Work out the finished part from the listing and answer in its coordinate system (mm). A direction names the side the tool comes from. Coordinates: 2 decimals unless noted, no trailing zeros. Loops run counter-clockwise (first coordinate to the right, second up) from the corner with the lowest first, then second, coordinate; pieces in that order, holes last. Notation, with made-up numbers: M 50.5,69 L 102.5,69 A14 ccw 102.5,93 Z; hole C -1,27 d8. An arc over 180 degrees is marked long. Write each question's results on one line, items separated by ' | '.
```python
from build123d import *

# Parameters (mm, degrees)
ESBO_O1_W                = 69
ESBO_O1_H                = 31.5
RESSALTO_EXTRUS_O1_DEPTH = 6
ESBO_O2_W                = 5
ESBO_O2_H                = 20
RESSALTO_EXTRUS_O2_DEPTH = 20
ESBO_O3_W                = 5
ESBO_O3_H                = 8
CORTE_EXTRUS_O1_DEPTH    = 11
ESBO_O4_W                = 4
ESBO_O4_H                = 31.5
RESSALTO_EXTRUS_O3_DEPTH = 20
ESBO_O5_W                = 16
ESBO_O5_H                = 8
CORTE_EXTRUS_O2_DEPTH    = 4
ESBO_O6_W                = 4
ESBO_O6_H                = 31.5
RESSALTO_EXTRUS_O4_DEPTH = 50
ESBO_O18_R               = 3.8
CORTE_EXTRUS_O3_DEPTH    = 4
ESBO_O19_R               = 5.8
CORTE_EXTRUS_O5_DEPTH    = 4
ESBO_O20_W               = 20
ESBO_O20_H               = 45
RESSALTO_EXTRUS_O9_DEPTH = 7
ESBO_O21_W               = 13
ESBO_O21_H               = 15
CORTE_EXTRUS_O6_DEPTH    = 7.7
ESBO_O22_W               = 13
ESBO_O22_H               = 20
CORTE_EXTRUS_O7_DEPTH    = 7.7
CORTE_EXTRUS_O9_DEPTH    = 3


with BuildPart() as part:
    # Esboço1 → Ressalto-extrusão1 (new body)
    with BuildSketch(Plane.XY):
        with Locations((-34.5, -15.931977108)):
            Rectangle(ESBO_O1_W, ESBO_O1_H)
    extrude(amount=RESSALTO_EXTRUS_O1_DEPTH)

    # Esboço2 → Ressalto-extrusão2 (add)
    with BuildSketch(Plane.XY.offset(6)):
        with Locations((-60, -21.681977108)):
            Rectangle(ESBO_O2_W, ESBO_O2_H)
    extrude(amount=RESSALTO_EXTRUS_O2_DEPTH)

    # Esboço3 → Corte-extrusão1 (cut)
    with BuildSketch(Plane.XY.offset(26)):
        with Locations((-60, -21.681977108)):
            Rectangle(ESBO_O3_W, ESBO_O3_H)
    extrude(amount=-CORTE_EXTRUS_O1_DEPTH, mode=Mode.SUBTRACT)

    # Esboço4 → Ressalto-extrusão3 (add)
    with BuildSketch(Plane.XY.offset(6)):
        with Locations((-52, -15.931977108)):
            Rectangle(ESBO_O4_W, ESBO_O4_H)
    extrude(amount=RESSALTO_EXTRUS_O3_DEPTH)

    # Esboço5 → Corte-extrusão2 (cut)
    with BuildSketch(Plane(origin=(-50, 0, 0), x_dir=(0, 0, -1), z_dir=(1, 0, 0))):
        with Locations((-14, -21.681977108)):
            Rectangle(ESBO_O5_W, ESBO_O5_H)
    extrude(amount=-CORTE_EXTRUS_O2_DEPTH, mode=Mode.SUBTRACT)

    # Esboço6 → Ressalto-extrusão4 (add)
    with BuildSketch(Plane(origin=(-50, 0, 0), x_dir=(0, 0, -1), z_dir=(1, 0, 0))):
        with Locations((-24, -15.931977108)):
            Rectangle(ESBO_O6_W, ESBO_O6_H)
    extrude(amount=RESSALTO_EXTRUS_O4_DEPTH)

    # Espelhar10: part across plane


with BuildPart() as part_1:
    add(part.part)
    add(part.part.mirror(Plane.ZX.offset(-0.181977108)))

    # Espelhar11: part across plane


with BuildPart() as part_2:
    add(part_1.part)
    add(part_1.part.mirror(Plane(origin=(0, 0, 0), x_dir=(0, 0, 1), z_dir=(1, 0, 0))))

    # Esboço18 → Corte-extrusão3 (cut)
    with BuildSketch(Plane.ZY.offset(54)):
        with Locations((16, -0.181977108)):
            Circle(ESBO_O18_R)
    extrude(amount=-CORTE_EXTRUS_O3_DEPTH, mode=Mode.SUBTRACT)

    # Esboço19 → Corte-extrusão5 (cut)
    with BuildSketch(Plane.XY.offset(26)):
        with Locations((35, 20.318022892)):
            Circle(ESBO_O19_R)
    extrude(amount=-CORTE_EXTRUS_O5_DEPTH, mode=Mode.SUBTRACT)

    # Esboço20 → Ressalto-extrusão9 (add)
    with BuildSketch(Plane(origin=(0, 0, 22), x_dir=(-1, 0, 0), z_dir=(0, 0, -1))):
        with Locations((34, -0.181977108)):
            Rectangle(ESBO_O20_W, ESBO_O20_H)
    extrude(amount=RESSALTO_EXTRUS_O9_DEPTH)

    # Esboço21 → Corte-extrusão6 (cut)
    with BuildSketch(Plane.XY.offset(26)):
        with Locations((-34, -12.181977108)):
            Rectangle(ESBO_O21_W, ESBO_O21_H)
    extrude(amount=-CORTE_EXTRUS_O6_DEPTH, mode=Mode.SUBTRACT)

    # Esboço22 → Corte-extrusão7 (cut)
    with BuildSketch(Plane.XY.offset(26)):
        with Locations((-34, 8.318022892)):
            Rectangle(ESBO_O22_W, ESBO_O22_H)
    extrude(amount=-CORTE_EXTRUS_O7_DEPTH, mode=Mode.SUBTRACT)

    # Esboço23 → Corte-extrusão9 (cut)
    with BuildSketch(Plane(origin=(0, -1.681977108, 0), x_dir=(1, 0, 0), z_dir=(0, 1, 0))):
        with BuildLine():
            Line((-31, -26), (-31, -22.15))
            ThreePointArc((-31, -22.15), (-34, -19.15), (-37, -22.15))
            Line((-37, -22.15), (-37, -26))
            Line((-37, -26), (-31, -26))
        make_face()
    extrude(amount=-CORTE_EXTRUS_O9_DEPTH, mode=Mode.SUBTRACT)


solid = part_2.part
```
1) Find section B-B, the plane x = 35. Give the vertices of the cut face in (y, z), and give its area (3 significant figures).
Check result:
outline: M -31.68,0 L 31.32,0 L 31.32,6 L -31.68,6 Z; M -31.68,22 L 14.52,22 L 14.52,26 L -31.68,26 Z; M 26.12,22 L 31.32,22 L 31.32,26 L 26.12,26 Z | area: 584 mm^2
2) Which of the six approach directions +Z, -Z, +X, -X, +Y, -Y give full straight-line access (tool end or side, diameter ignored) to faces 4 (the face through (-60, 17.318, 21)), 5 (the face through (-40.5, -12, 22)), 6 (the face through (54, 0, 16)), 7 (the face through (60, 21, 15)), 8 (the face through (-62.5, 21, 14))?
Check result:
face 4: +Z, -X | face 5: +Z | face 6: +Z, +Y, -Y | face 7: +Z, +X | face 8: +Z, -X, +Y, -Y
3) For a pull along Z with two mould halves and no side action, classify faces 1 (the face through (-37, -3, 24)), 2 (the face through (60, -15, 26)), 3 (the face through (50, 0, 14)) as released by +Z, released by -Z, zero draft, split by the parting line, or undercut.
Check result:
face 1: zero draft | face 2: released by +Z | face 3: undercut
4) Find section C-C, the plane z = 8.5. Give the number of separate pieces and of enclosed holes in the cut face, and give its area (3 significant figures).
Check result:
separate pieces: 10 | enclosed holes: 0 | area: 776 mm^2
5) Find section D-D, the plane x = -12. Give the vertices of the cut face in (y, z).
Check result:
outline: M -31.68,0 L 31.32,0 L 31.32,6 L -31.68,6 Z; M -31.68,22 L 31.32,22 L 31.32,26 L -31.68,26 Z
6) Given pin 1 Ø4 at (y, z) = (14, 11) entering from +X; pin 2 Ø12 at (y, z) = (14, 19.5) entering from -X; pin 3 Ø5.5 at (x, y) = (-60.5, 22) entering from +Z, each flat-ended and moving along its own axis, determine where each tip first touches the part or whether it passes through.
Check result:
pin 1: x = 62.5 | pin 2: x = -62.5 | pin 3: z = 15
7) Straight lines are drawn through the part: probe 1 along X at (y, z) = (10, 15.75); probe 2 along Y at (x, z) = (-51.1, 16); probe 3 along X at (y, z) = (0.5, 19). For each, find the intervals that lie inside material, in ascending order. Write a range as [from, to].
Check result:
probe 1: [-54, -50], [-44, -24], [50, 54] | probe 2: [-31.68, -25.68], [-17.68, -3.98], [3.62, 17.32], [25.32, 31.32] | probe 3: [-44, -40.5], [-27.5, -24], [50, 54]
8) Find section A-A, the plane x = -34. Give the vertices of the cut face in (y, z), and give its area (3 significant figures).
Check result:
outline: M -31.68,0 L 31.32,0 L 31.32,6 L -31.68,6 Z; M -31.68,22 L -22.68,22 L -22.68,15 L 22.32,15 L 22.32,22 L 31.32,22 L 31.32,26 L 18.32,26 L 18.32,18.3 L -1.68,18.3 L -1.68,19.15 L -4.68,19.15 L -4.68,18.3 L -19.68,18.3 L -19.68,26 L -31.68,26 Z | area: 655 mm^2
